The model under review builds one solid part; all positions refer to its coordinate system, in mm. Face numbers are marked on the shaded views. A direction names the side the tool comes from. Coordinates: 2 decimals unless noted, no trailing zeros. Write each loop counter-clockwise with the first axis right and the second up, starting at its lowest first coordinate (ties: lowest second). Pieces come first, ordered by that corner, then holes. Notation, with made-up numbers: (10, 49.25) -> (43, 49.25) arc R25 cw to (43, 67.25) -> close; hole circle Ø5 at (5.25, 11.25). An arc over 180 degrees is marked (long way). Put each result on its own line as item: value. Start each with the question number.
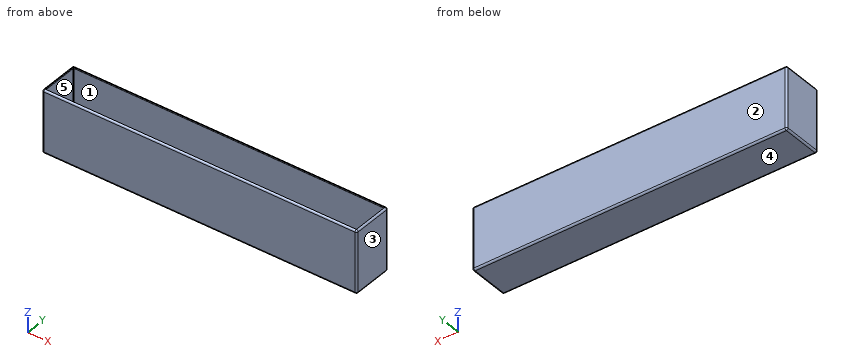
from build123d import *

# Parameters (mm, degrees)
F0_W     = 685.8
F0_H     = 136.525
F1_DEPTH = 88.9
F2_R     = 3.81
F3_T     = -2.54


# Not quite as in the source:
# - a shell that OpenCascade refuses in one call is made with other operations: the cavity is built on its own and cut out


with BuildPart() as f1:
    # F0 (on Front) → F1 (new body)
    with BuildSketch(Plane.XZ):
        Rectangle(F0_W, F0_H)
    extrude(amount=F1_DEPTH)

    # F2
    f2_edges = [f1.edges().sort_by_distance(p)[0] for p in [
        (-342.9, -44.45, 68.2625),
        (342.9, -44.45, 68.2625),
        (0, 0, 68.2625),
        (0, -88.9, 68.2625),
        (-342.9, 0, 0),
        (0, 0, -68.2625),
        (342.9, 0, 0),
        (-342.9, -44.45, -68.2625),
        (-342.9, -88.9, 0),
        (0, -88.9, -68.2625),
        (342.9, -88.9, 0),
        (342.9, -44.45, -68.2625),
    ]]
    fillet(f2_edges, radius=F2_R)

    # F3: a shell. OpenCascade refuses it in one call, so the cavity is built on its own and cut out:
    # the body offset inwards by the wall thickness, plus a prism from it out through each open face.
    f3_core = offset(f1.part, amount=F3_T, mode=Mode.PRIVATE)
    f3_exits = [f3_core.faces().sort_by_distance(p)[0] for p in [
        (0, -44.45, 65.7225),
    ]]
    add(f3_core, mode=Mode.SUBTRACT)
    extrude(f3_exits, amount=-F3_T, mode=Mode.SUBTRACT)


solid = f1.part
1. Consider section A-A on z = -45. State the section outline as (x, y) points.
2. Insertion check: P1, Ø1.5, axis at x = 153.5, y = -21.5, coming from the +Z side; P2, Ø1.3, axis at y = -60.5, z = 66.5, coming from the -X side; P3, Ø0.8, axis at x = -61, z = 67.5, coming from the +Y side. Each pin has a flat end and moves straight along its axis. Give the tip position at first contact, or say it passes through.
3. Wall thickness on line 1 (Y direction, x = -110, z = -61); line 2 (X direction, y = -36.5, z = 33.5); line 3 (Z direction, x = 6.5, y = -75): over which ranges is each line inside the solid? List them lowest first. Write a range as from..to.
4. Consider section C-C on y = -65.5. State the section outline as (x, z) points, then the cut area to 3 significant figures.
5. The part is to be moulded in two halves that separate along Z. For the marked faces 3, 4 and 5, say which applies: released by +Z, released by -Z, zero draft, split by the parting line, or undercut.
6. Tool access review of the marked faces 1 and 2: name each direction out of +Z, -Z, +X, -X, +Y, -Y from which nothing blocks a thin tool from reaching the whole face with its end or side.
7. Consider section B-B on x = 80.5. State the section outline as (y, z) points, then the cut area to 3 significant figures.
Output values:
1. outline: (-342.9, -85.09) arc R3.81 ccw to (-339.09, -88.9) -> (339.09, -88.9) arc R3.81 ccw to (342.9, -85.09) -> (342.9, -3.81) arc R3.81 ccw to (339.09, 0) -> (-339.09, 0) arc R3.81 ccw to (-342.9, -3.81) -> close; hole (-340.36, -85.09) arc R1.27 ccw to (-339.09, -86.36) -> (339.09, -86.36) arc R1.27 ccw to (340.36, -85.09) -> (340.36, -3.81) arc R1.27 ccw to (339.09, -2.54) -> (-339.09, -2.54) arc R1.27 ccw to (-340.36, -3.81) -> close
2. P1: stops at z = -65.72
2. P2: stops at x = -342.63
2. P3: stops at y = -1.07
3. line 1: y = -88.9..-86.36, -2.54..0
3. line 2: x = -342.9..-340.36, 340.36..342.9
3. line 3: z = -68.26..-65.72
4. outline: (-342.9, -64.45) arc R3.81 ccw to (-339.09, -68.26) -> (339.09, -68.26) arc R3.81 ccw to (342.9, -64.45) -> (342.9, 64.45) arc R3.81 ccw to (339.09, 68.26) -> (339.09, 65.72) arc R1.27 cw to (340.36, 64.45) -> (340.36, -64.45) arc R1.27 cw to (339.09, -65.72) -> (-339.09, -65.72) arc R1.27 cw to (-340.36, -64.45) -> (-340.36, 64.45) arc R1.27 cw to (-339.09, 65.72) -> (-339.09, 68.26) arc R3.81 ccw to (-342.9, 64.45) -> close
4. area: 2,420 mm^2
5. face 3: zero draft
5. face 4: released by -Z
5. face 5: undercut
6. face 1: none
6. face 2: +Z, -Z, +X, -X, +Y
7. outline: (-88.9, -64.45) arc R3.81 ccw to (-85.09, -68.26) -> (-3.81, -68.26) arc R3.81 ccw to (0, -64.45) -> (0, 64.45) arc R3.81 ccw to (-3.81, 68.26) -> (-3.81, 65.72) arc R1.27 cw to (-2.54, 64.45) -> (-2.54, -64.45) arc R1.27 cw to (-3.81, -65.72) -> (-85.09, -65.72) arc R1.27 cw to (-86.36, -64.45) -> (-86.36, 64.45) arc R1.27 cw to (-85.09, 65.72) -> (-85.09, 68.26) arc R3.81 ccw to (-88.9, 64.45) -> close
7. area: 902 mm^2
